from build123d import *

# Parameters (mm, degrees)
SKETCH_1_R          = 19.55
EXTRUDE_1_DEPTH     = 7
SKETCH_2_R          = 10.6
EXTRUDE_2_DEPTH     = 12
FILLET_1_R          = 0.5
SKETCH_3_R          = 4
CUT_EXTRUDE_3_DEPTH = 34.547056503
SKETCH_4_R          = 2
CUT_EXTRUDE_4_DEPTH = 31.139757796


with BuildPart() as part:
    # Эскиз1 → Вытянуть1 (new body)
    with BuildSketch(Plane.XY):
        Circle(SKETCH_1_R)
    extrude(amount=EXTRUDE_1_DEPTH)

    # Эскиз2 → Вытянуть2 (add)
    with BuildSketch(Plane.XY.offset(7)):
        Circle(SKETCH_2_R)
    extrude(amount=EXTRUDE_2_DEPTH)

    # Скругление1
    fillet_1_edges = [part.edges().sort_by_distance(p)[0] for p in [
        (-10.6, 0, 7),
    ]]
    fillet(fillet_1_edges, radius=FILLET_1_R)

    # Эскиз3 → Вытянуть3 (cut, through all)
    with BuildSketch(Plane.XY.offset(19)):
        Circle(SKETCH_3_R)
    extrude(amount=-CUT_EXTRUDE_3_DEPTH, mode=Mode.SUBTRACT)

    # Эскиз4 → Вытянуть4 (cut, through all)
    with BuildSketch(Plane.XY.offset(7)):
        with Locations((0, 15.4)):
            Circle(SKETCH_4_R)
        with Locations((14.646270351, 4.758861713)):
            Circle(SKETCH_4_R)
        with Locations((9.051892885, -12.458861713)):
            Circle(SKETCH_4_R)
        with Locations((-9.051892885, -12.458861713)):
            Circle(SKETCH_4_R)
        with Locations((-14.646270351, 4.758861713)):
            Circle(SKETCH_4_R)
    extrude(amount=-CUT_EXTRUDE_4_DEPTH, mode=Mode.SUBTRACT)


solid = part.part
Can you work these out from the model? Positions are in its coordinate system, mm. A direction names the side the tool comes from. Give positions to 0.01 mm unless a question says otherwise; leave off trailing zeros. Order: outer loops, then holes, each group sorted by start corner. A loop starts at its lowest first (then second) coordinate and runs counter-clockwise, first axis right, second up. Notation, with made-up numbers: M 49,59 L 104,59 A35 cw 104,94 Z; hole C 32.25,18 d8. An arc over 180 degrees is marked long. One line per item, written item: value.
Item 1: If we mould it in two halves opening along X, with no side actions, what happens to faces 1 (the face through (5, 0, 19)), 2 (the face through (-0.867, -3.905, 9.633)), 3 (the face through (18.65, 5.87, 3.45))? For each: pulls with the +X half, pulls with the -X half, needs draft (parallel to the pull), parting line crosses it, or undercut.
Verdict:
face 1: needs draft
face 2: undercut
face 3: parting line crosses it
Item 2: Please list where these lines run through material, in increasing order: line 1 (Z direction, x = 12, y = 4); line 2 (X direction, y = 6.5, z = 4.25); line 3 (X direction, y = 14, z = 2).
Verdict:
line 1: 0 to 7
line 2: -18.44 to -15.63, -13.66 to 13.66, 15.63 to 18.44
line 3: -13.65 to -1.43, 1.43 to 13.65
Item 3: For pin 1 (10 mm diameter, centred on y = -0.5, z = 15.5, fed in from -X); pin 2 (3 mm diameter, centred on x = -6, z = 3.5, fed in from +Y); pin 3 (1.5 mm diameter, centred on x = -9.5, z = 5, fed in from +Y), each with a flat end and sliding along its axis, tell me the tip position at first contact or that it passes through.
Verdict:
pin 1: x = -10.6
pin 2: y = 19.03
pin 3: y = 17.48
Item 4: If we section it at A-A on x = 0: Write out the boundary of the cut face in (y, z).
Verdict:
outline: M -19.55,0 L -4,0 L -4,19 L -10.6,19 L -10.6,7.5 A0.5 cw -11.1,7 L -19.55,7 Z; M 4,0 L 13.4,0 L 13.4,7 L 11.1,7 A0.5 cw 10.6,7.5 L 10.6,19 L 4,19 Z; M 17.4,0 L 19.55,0 L 19.55,7 L 17.4,7 Z
Item 5: For faces 4 (the face through (9.79, -4.06, 13.17)), 5 (the face through (1.075, 17.086, 3.549)), which set-ups out of +Z, -Z, +X, -X, +Y, -Y let a thin tool reach every point of the face, with its end or its side?
Verdict:
face 4: +Z
face 5: +Z, -Z
Item 6: If we section it at C-C on z = 17.25: Write out the boundary of the cut face in (x, y).
Verdict:
outline: C 0,0 d21.2; hole C 0,0 d8
Item 7: If we section it at D-D on x = 15: Write out the boundary of the cut face in (y, z).
Verdict:
outline: M -12.54,0 L 2.79,0 L 2.79,7 L -12.54,7 Z; M 6.73,0 L 12.54,0 L 12.54,7 L 6.73,7 Z
Item 8: If we section it at B-B on y = 0: Write out the boundary of the cut face in (x, z).
Verdict:
outline: M -19.55,0 L -4,0 L -4,19 L -10.6,19 L -10.6,7.5 A0.5 cw -11.1,7 L -19.55,7 Z; M 4,0 L 19.55,0 L 19.55,7 L 11.1,7 A0.5 cw 10.6,7.5 L 10.6,19 L 4,19 Z
